```python
from build123d import *

# Parameters (mm, degrees)
SKETCH2_W           = 55
SKETCH2_H           = 56
SKETCH2_R           = 1.75
BOSS_EXTRUDE1_DEPTH = 5
SKETCH3_W           = 30
SKETCH3_H           = 20
BOSS_EXTRUDE2_DEPTH = 5
SKETCH5_W           = 10
SKETCH5_H           = 22
BOSS_EXTRUDE3_DEPTH = 5
SKETCH6_R           = 1.75
CUT_EXTRUDE1_DEPTH  = 5


with BuildPart() as part:
    # Sketch2 → Boss-Extrude1 (new body)
    with BuildSketch(Plane(origin=(0, 0, 0), x_dir=(1, 0, 0), z_dir=(0, 1, 0))):
        Rectangle(SKETCH2_W, SKETCH2_H)
        with Locations(Location((-20, 8, 0), (0, 0, 270))):
            Circle(SKETCH2_R, mode=Mode.SUBTRACT)
        with Locations(Location((-20, 23, 0), (0, 0, 270))):
            Circle(SKETCH2_R, mode=Mode.SUBTRACT)
        with Locations(Location((20, 8, 0), (0, 0, 90))):
            Circle(SKETCH2_R, mode=Mode.SUBTRACT)
        with Locations(Location((20, 23, 0), (0, 0, 90))):
            Circle(SKETCH2_R, mode=Mode.SUBTRACT)
        with Locations(Location((20, -8, 0), (0, 0, 270))):
            Circle(SKETCH2_R, mode=Mode.SUBTRACT)
        with Locations(Location((20, -23, 0), (0, 0, 270))):
            Circle(SKETCH2_R, mode=Mode.SUBTRACT)
        with Locations(Location((-20, -8, 0), (0, 0, 90))):
            Circle(SKETCH2_R, mode=Mode.SUBTRACT)
        with Locations(Location((-20, -23, 0), (0, 0, 90))):
            Circle(SKETCH2_R, mode=Mode.SUBTRACT)
    extrude(amount=BOSS_EXTRUDE1_DEPTH)

    # Sketch3 → Boss-Extrude2 (add)
    with BuildSketch(Plane(origin=(0, 5, 0), x_dir=(1, 0, 0), z_dir=(0, 1, 0))):
        Polygon((27.5, 28), (27.5, -28), (77.5, -28), (77.5, -16), (87.5, -16), (87.5, 6), (77.5, 6), (77.5, 18), align=None)
        with Locations((52.5, -5)):
            Rectangle(SKETCH3_W, SKETCH3_H, mode=Mode.SUBTRACT)
    extrude(amount=-BOSS_EXTRUDE2_DEPTH)

    # Sketch5 → Boss-Extrude3 (add)
    with BuildSketch(Plane(origin=(0, 5, 0), x_dir=(1, 0, 0), z_dir=(0, 1, 0))):
        with Locations((-32.5, -5)):
            Rectangle(SKETCH5_W, SKETCH5_H)
    extrude(amount=-BOSS_EXTRUDE3_DEPTH)

    # Sketch6 → Cut-Extrude1 (cut)
    with BuildSketch(Plane(origin=(0, 5, 0), x_dir=(1, 0, 0), z_dir=(0, 1, 0))):
        with Locations(Location((-7.5, 12, 0), (0, 0, 270))):
            Circle(SKETCH6_R)
        with Locations(Location((52.5, 12, 0), (0, 0, 270))):
            Circle(SKETCH6_R)
        with Locations(Location((52.5, -23, 0), (0, 0, 270))):
            Circle(SKETCH6_R)
    extrude(amount=-CUT_EXTRUDE1_DEPTH, mode=Mode.SUBTRACT)


solid = part.part
```
Can you work these out from the model? Positions are in its coordinate system, mm. A direction names the side the tool comes from. Give positions to 0.01 mm unless a question says otherwise; leave off trailing zeros. Loops run counter-clockwise (first coordinate to the right, second up) from the corner with the lowest first, then second, coordinate; pieces in that order, holes last. Notation, with made-up numbers: M 18,7 L 55,7 A15 ccw 55,12 Z; hole C 65.25,28 d4. An arc over 180 degrees is marked long. Answer in a Markdown table with one row per item.
1. If I drill on line 1 along X through (y, z) = (2.1, -8); line 2 along X through (y, z) = (3.85, 8); line 3 along X through (y, z) = (2.95, 23), over which ranges is the centre line in solid material (lowest first)?
Taken from the geometry:
| item | result |
|---|---|
| line 1 | x = -27.5 to -21.75, -18.25 to 18.25, 21.75 to 77.5 |
| line 2 | x = -37.5 to -21.75, -18.25 to 18.25, 21.75 to 37.5, 67.5 to 87.5 |
| line 3 | x = -27.5 to -21.75, -18.25 to 18.25, 21.75 to 50.75, 54.25 to 77.5 |
2. Thinking about a two-plate mould opening in Z: for faces 4 (the cylindrical face through (21.735, 2.465, 7.772)), 5 (the flat face through (77.5, 3, 22)), 6 (the flat face through (0, 2, -28)), which applies, released by +Z, released by -Z, zero draft, split by the parting line, or undercut?
Taken from the geometry:
| item | result |
|---|---|
| face 4 | undercut |
| face 5 | zero draft |
| face 6 | released by -Z |
3. Which directions (+Z, -Z, +X, -X, +Y, -Y) give clear straight access to the entire face, cutting with the end or side of a thin tool? Please do faces 1 (the flat face through (24, 0, 0)), 2 (the flat face through (52, 3, 15)), 3 (the flat face through (83, 3, -6)).
Taken from the geometry:
| item | result |
|---|---|
| face 1 | +Z, -Z, +X, -X, -Y |
| face 2 | +Y, -Y |
| face 3 | -Z, +X, +Y, -Y |
4. Suppose I cut it at B-B on x = -20. Write out the boundary of the cut face in (y, z).
Taken from the geometry:
| item | result |
|---|---|
| outline | M 0,-28 L 5,-28 L 5,-24.75 L 0,-24.75 Z; M 0,-21.25 L 5,-21.25 L 5,-9.75 L 0,-9.75 Z; M 0,-6.25 L 5,-6.25 L 5,6.25 L 0,6.25 Z; M 0,9.75 L 5,9.75 L 5,21.25 L 0,21.25 Z; M 0,24.75 L 5,24.75 L 5,28 L 0,28 Z |
5. Suppose I cut it at D-D on y = 1.9. Count the separate pieces of the cut face and the enclosed holes in it, plus the area to 3 significant figures.
Taken from the geometry:
| item | result |
|---|---|
| separate pieces | 1 |
| enclosed holes | 12 |
| area | 5,360 mm² |
6. For pin 1 Ø2 at (x, z) = (-7.5, -12) entering from -Y; pin 2 Ø2.5 at (y, z) = (2, -19.5) entering from -X, each with a flat end and sliding along its axis, tell me the tip position at first contact or that it passes through.
Taken from the geometry:
| item | result |
|---|---|
| pin 1 | passes through |
| pin 2 | stops at x = -27.5 |
7. Suppose I cut it at C-C on z = -23. Write out the boundary of the cut face in (x, y).
Taken from the geometry:
| item | result |
|---|---|
| outline | M -27.5,0 L -21.75,0 L -21.75,5 L -27.5,5 Z; M -18.25,0 L 18.25,0 L 18.25,5 L -18.25,5 Z; M 21.75,0 L 52.5,0 L 52.5,5 L 21.75,5 Z |
8. Suppose I cut it at A-A on z = 23. Write out the boundary of the cut face in (x, y), plus the area to 4 significant figures.
Taken from the geometry:
| item | result |
|---|---|
| outline | M -27.5,0 L -21.75,0 L -21.75,5 L -27.5,5 Z; M -18.25,0 L 18.25,0 L 18.25,5 L -18.25,5 Z; M 21.75,0 L 50.75,0 L 50.75,5 L 21.75,5 Z; M 54.25,0 L 77.5,0 L 77.5,5 L 54.25,5 Z |
| area | 472.5 mm² |
